```python
from build123d import *

# Parameters (mm, degrees)
SKETCH1_W               = 42.62295082
SKETCH1_H               = 50
SKETCH1_R               = 2.677018134
BOSS_EXTRUDE1_DEPTH     = 20
SKETCH2_R               = 11
CUT_EXTRUDE2_DEPTH      = 11
SKETCH3_R               = 1.75
CUT_EXTRUDE3_DEPTH      = 10
CUT_EXTRUDE6_START      = -5
CUT_EXTRUDE6_DEPTH      = 34.460095998
SKETCH30_W              = 42.62295082
SKETCH30_H              = 20
BOSS_EXTRUDE8_DEPTH     = 20.23
SKETCH10_W              = 42.62295082
SKETCH10_H              = 16
BOSS_EXTRUDE2_DEPTH     = 20
SKETCH14_W              = 6
SKETCH14_H              = 13
CUT_EXTRUDE7_DEPTH      = 78.238778062
BOSS_EXTRUDE3_DEPTH     = 8
CUT_EXTRUDE9_DEPTH      = 8
SKETCH18_W              = 0.9
SKETCH18_H              = 4
SKETCH18_W_2            = 1.8
CUT_EXTRUDE10_DEPTH     = 10.2
CUT_EXTRUDE8_DEPTH      = 71.769170482
CUT_EXTRUDE8_DEPTH_BACK = 71.769170482
SKETCH15_R              = 1
CUT_EXTRUDE5_DEPTH      = 82.374415455
CUT_EXTRUDE5_DEPTH_BACK = 50
SKETCH6_W               = 9.034037672
SKETCH6_H               = 5.5
SKETCH20_W              = 8
SKETCH20_H              = 20
BOSS_EXTRUDE5_DEPTH     = 13
SKETCH21_W              = 8
SKETCH21_H              = 6
CUT_EXTRUDE11_DEPTH     = 13
SKETCH22_R              = 1
CUT_EXTRUDE12_DEPTH     = 71.769170482
SKETCH24_W              = 50.62295082
SKETCH24_H              = 5
BOSS_EXTRUDE6_DEPTH     = 15
SKETCH25_W              = 50.62295082
SKETCH25_H              = 15
BOSS_EXTRUDE7_DEPTH     = 15
SKETCH26_R              = 1
CUT_EXTRUDE13_DEPTH     = 10
SKETCH27_W              = 4
SKETCH27_H              = 1.8
CUT_EXTRUDE14_DEPTH     = 10.2
SKETCH29_W              = 20
SKETCH29_H              = 3.2
CUT_EXTRUDE15_DEPTH     = 9


with BuildPart() as part:
    # Sketch1 → Boss-Extrude1 (new body)
    with BuildSketch(Plane.XY):
        Rectangle(SKETCH1_W, SKETCH1_H)
        with Locations((-13, -15.25)):
            Circle(SKETCH1_R, mode=Mode.SUBTRACT)
        with Locations(Location((13, -15.25, 0), (0, 0, 180))):
            Circle(SKETCH1_R, mode=Mode.SUBTRACT)
        with Locations((13, 15.25)):
            Circle(SKETCH1_R, mode=Mode.SUBTRACT)
        with Locations(Location((-13, 15.25, 0), (0, 0, 180))):
            Circle(SKETCH1_R, mode=Mode.SUBTRACT)
    extrude(amount=BOSS_EXTRUDE1_DEPTH)

    # Sketch2 → Cut-Extrude2 (cut)
    with BuildSketch(Plane.XY):
        Circle(SKETCH2_R)
    extrude(amount=CUT_EXTRUDE2_DEPTH, mode=Mode.SUBTRACT)

    # Sketch3 → Cut-Extrude3 (cut)
    with BuildSketch(Plane(origin=(0, 0, 0), x_dir=(-1, 0, 0), z_dir=(0, 0, -1))):
        with Locations((-15, 0)):
            Circle(SKETCH3_R)
        with Locations(Location((15, 0, 0), (0, 0, 180))):
            Circle(SKETCH3_R)
    extrude(amount=-CUT_EXTRUDE3_DEPTH, mode=Mode.SUBTRACT)

    # Sketch9 → Cut-Extrude6 (cut, through all)
    with BuildSketch(Plane(origin=(0, 0, 0), x_dir=(-1, 0, 0), z_dir=(0, 0, -1)).offset(CUT_EXTRUDE6_START)):
        Polygon((-15, 3.175426481), (-17.75, 1.58771324), (-17.75, -1.58771324), (-15, -3.175426481), (-12.25, -1.58771324), (-12.25, 1.58771324), align=None)
        Polygon((12.25, 1.58771324), (15, 3.175426481), (17.75, 1.58771324), (17.75, -1.58771324), (15, -3.175426481), (12.25, -1.58771324), align=None)
    extrude(amount=-CUT_EXTRUDE6_DEPTH, mode=Mode.SUBTRACT)

    # Sketch30 → Boss-Extrude8 (add)
    with BuildSketch(Plane.XZ.offset(25)):
        with Locations((0, 10)):
            Rectangle(SKETCH30_W, SKETCH30_H)
    extrude(amount=BOSS_EXTRUDE8_DEPTH)

    # Sketch10 → Boss-Extrude2 (add)
    with BuildSketch(Plane.XY):
        with Locations((0, -53.23)):
            Rectangle(SKETCH10_W, SKETCH10_H)
    extrude(amount=BOSS_EXTRUDE2_DEPTH)

    # Sketch14 → Cut-Extrude7 (cut, through all)
    with BuildSketch(Plane.ZY.offset(21.31147541)):
        with Locations((8, -54.73)):
            Rectangle(SKETCH14_W, SKETCH14_H)
    extrude(amount=-CUT_EXTRUDE7_DEPTH, mode=Mode.SUBTRACT)

    # Sketch16 → Boss-Extrude3 (add)
    with BuildSketch(Plane(origin=(21.31147541, 0, 0), x_dir=(0, 0, -1), z_dir=(1, 0, 0))):
        Polygon((-10, 25), (-10, -48.23), (-5, -48.23), (0, -48.23), (0, 25), align=None)
        Polygon((-11, -48.23), (-10, -48.23), (-10, 25), (-20, 25), (-20, -48.23), align=None)
    extrude(amount=BOSS_EXTRUDE3_DEPTH)

    # Sketch17 → Cut-Extrude9 (cut)
    with BuildSketch(Plane(origin=(29.31147541, 0, 0), x_dir=(0, 0, -1), z_dir=(1, 0, 0))):
        with BuildLine():
            ThreePointArc((-10, 7.56), (-11.175, 6.385), (-10, 5.21))
            Line((-10, 5.21), (-10, 7.56))
        make_face()
        with BuildLine():
            Line((-10, 7.56), (-10, 5.21))
            ThreePointArc((-10, 5.21), (-9.169149532, 5.554149532), (-8.825, 6.385))
            ThreePointArc((-8.825, 6.385), (-9.169149532, 7.215850468), (-10, 7.56))
        make_face()
        with BuildLine():
            ThreePointArc((-10, -28.44), (-11.175, -29.615), (-10, -30.79))
            Line((-10, -30.79), (-10, -28.44))
        make_face()
        with BuildLine():
            Line((-10, -28.44), (-10, -30.79))
            ThreePointArc((-10, -30.79), (-9.169149532, -30.445850468), (-8.825, -29.615))
            ThreePointArc((-8.825, -29.615), (-9.169149532, -28.784149532), (-10, -28.44))
        make_face()
    extrude(amount=-CUT_EXTRUDE9_DEPTH, mode=Mode.SUBTRACT)

    # Sketch18 → Cut-Extrude10 (cut)
    with BuildSketch(Plane(origin=(0, 0, 0), x_dir=(-1, 0, 0), z_dir=(0, 0, -1))):
        with Locations((-24.86147541, 6.385)):
            Rectangle(SKETCH18_W, SKETCH18_H)
        with Locations((-25.76147541, 6.385)):
            Rectangle(SKETCH18_W, SKETCH18_H)
        with Locations((-25.31147541, -29.615)):
            Rectangle(SKETCH18_W_2, SKETCH18_H)
    extrude(amount=-CUT_EXTRUDE10_DEPTH, mode=Mode.SUBTRACT)

    # Sketch15 → Cut-Extrude8 (cut, two sides: drawn at the far end of the back side and taken through both)
    with BuildSketch(Plane(origin=(0, 0, 0), x_dir=(-1, 0, 0), z_dir=(0, 0, -1)).offset(-CUT_EXTRUDE8_DEPTH_BACK)):
        with Locations(Location((16.31147541, -58.03, 0), (0, 0, 180))):
            Circle(SKETCH15_R)
        with Locations((16.31147541, -51.43)):
            Circle(SKETCH15_R)
    extrude(amount=CUT_EXTRUDE8_DEPTH + CUT_EXTRUDE8_DEPTH_BACK, mode=Mode.SUBTRACT)

    # Sketch6 → Cut-Extrude5 (cut, two sides: drawn at the far end of the back side and taken through both)
    with BuildSketch(Plane.XZ.offset(48.23).offset(-CUT_EXTRUDE5_DEPTH_BACK)):
        with Locations((0, 13.75)):
            Rectangle(SKETCH6_W, SKETCH6_H)
    extrude(amount=CUT_EXTRUDE5_DEPTH + CUT_EXTRUDE5_DEPTH_BACK, mode=Mode.SUBTRACT)

    # Sketch20 → Boss-Extrude5 (add)
    with BuildSketch(Plane(origin=(0, -48.23, 0), x_dir=(-1, 0, 0), z_dir=(0, -1, 0))):
        with Locations((-25.31147541, -10)):
            Rectangle(SKETCH20_W, SKETCH20_H)
    extrude(amount=BOSS_EXTRUDE5_DEPTH)

    # Sketch21 → Cut-Extrude11 (cut)
    with BuildSketch(Plane(origin=(0, -61.23, 0), x_dir=(-1, 0, 0), z_dir=(0, -1, 0))):
        with Locations((-25.31147541, -8)):
            Rectangle(SKETCH21_W, SKETCH21_H)
    extrude(amount=-CUT_EXTRUDE11_DEPTH, mode=Mode.SUBTRACT)

    # Sketch22 → Cut-Extrude12 (cut, through all)
    with BuildSketch(Plane(origin=(0, 0, 0), x_dir=(-1, 0, 0), z_dir=(0, 0, -1))):
        with Locations((-24.31147541, -58.03)):
            Circle(SKETCH22_R)
        with Locations((-24.31147541, -51.43)):
            Circle(SKETCH22_R)
    extrude(amount=-CUT_EXTRUDE12_DEPTH, mode=Mode.SUBTRACT)

    # Sketch24 → Boss-Extrude6 (add)
    with BuildSketch(Plane.XZ.offset(61.23)):
        with Locations((4, 2.5)):
            Rectangle(SKETCH24_W, SKETCH24_H)
    extrude(amount=BOSS_EXTRUDE6_DEPTH)

    # Sketch25 → Boss-Extrude7 (add)
    with BuildSketch(Plane.XY.offset(5)):
        with Locations((4, -68.73)):
            Rectangle(SKETCH25_W, SKETCH25_H)
    extrude(amount=BOSS_EXTRUDE7_DEPTH)

    # Sketch26 → Cut-Extrude13 (cut)
    with BuildSketch(Plane.XZ.offset(76.23)):
        with BuildLine():
            ThreePointArc((-15, 10), (-14, 9), (-13, 10))
            Line((-13, 10), (-15, 10))
        make_face()
        with BuildLine():
            Line((-15, 10), (-13, 10))
            ThreePointArc((-13, 10), (-14, 11), (-15, 10))
        make_face()
        with Locations(Location((22, 10, 0), (0, 0, 270))):
            Circle(SKETCH26_R)
    extrude(amount=-CUT_EXTRUDE13_DEPTH, mode=Mode.SUBTRACT)

    # Sketch27 → Cut-Extrude14 (cut)
    with BuildSketch(Plane(origin=(0, 0, 0), x_dir=(-1, 0, 0), z_dir=(0, 0, -1))):
        with Locations((-22.00147541, -72.23)):
            Rectangle(SKETCH27_W, SKETCH27_H)
        with Locations((14.00147541, -72.23)):
            Rectangle(SKETCH27_W, SKETCH27_H)
    extrude(amount=-CUT_EXTRUDE14_DEPTH, mode=Mode.SUBTRACT)

    # Sketch29 → Cut-Extrude15 (cut)
    with BuildSketch(Plane.XY.offset(20)):
        with Locations((4, -49.83)):
            Rectangle(SKETCH29_W, SKETCH29_H)
        Polygon((-6, -51.43), (-6, -53.105302663), (4, -54.73), (14, -53.105302663), (14, -51.43), align=None)
        Polygon((4, -54.73), (-6, -53.105302663), (-6, -56.354697337), align=None)
        with Locations((4, -59.63)):
            Rectangle(SKETCH29_W, SKETCH29_H)
        Polygon((14, -56.354697337), (4, -54.73), (-6, -56.354697337), (-6, -58.03), (14, -58.03), align=None)
        Polygon((14, -53.105302663), (4, -54.73), (14, -56.354697337), align=None)
    extrude(amount=-CUT_EXTRUDE15_DEPTH, mode=Mode.SUBTRACT)


solid = part.part
```
Geometry: final body of the model. Coordinates: model frame, mm. A direction names the side the tool comes from. Coordinates: 2 decimals unless noted, no trailing zeros. Order: outer loops, then holes, each group sorted by start corner. A loop starts at its lowest first (then second) coordinate and runs counter-clockwise, first axis right, second up. Notation, with made-up numbers: (24.5, 17.5) -> (78.5, 17.5) arc R28 cw to (78.5, 43.5) -> close; hole circle Ø3 at (-6, 61.25). An arc over 180 degrees is marked (long way). Write each question's results on one line, items separated by ' | '. Start each with the question number.
1) Set-up query: faces 3 (the cylindrical face through (-13.46, -71.3, 10.84)), 4 (the flat face through (22, -71.33, 5)), 5 (the flat face through (12.25, 0, 12)). Return all of +Z, -Z, +X, -X, +Y, -Y with unobstructed straight access to the full face (end or side cutting, diameter ignored); none if empty.
2) First-contact query: pin 1 (0.5 mm diameter, centred on x = 21, y = -72.5, fed in from -Z). Flat tip, straight axial feed; report the tip coordinate or a pass-through.
3) Mould query, pull axis Y, two halves, no side actions, for faces 1 (the flat face through (0, 3, 11)), 2 (the flat face through (29.311, -26, 10)). Classes: released by +Y, released by -Y, zero draft, split by the parting line, or undercut.
4) Cut plane C-C, the plane y = -39. Output: boundary loops of the cut face in (x, z).
5) Material intervals for line 1 along Y through (x, z) = (13, 2.5); line 2 along Y through (x, z) = (-13, 7.5); line 3 along Z through (x, y) = (-0.5, -31), sorted ascending.
6) Cut plane B-B, the plane x = 0. Output: boundary loops of the cut face in (y, z).
7) Cut plane A-A, the plane z = 2.25. State how many separate pieces and enclosed holes the cut face has, and give its area (3 significant figures).
Checks:
1) face 3: -Y | face 4: -Z | face 5: +Z
2) pin 1: z = 10.2
3) face 1: undercut | face 2: zero draft
4) outline: (-21.31, 0) -> (29.31, 0) -> (29.31, 20) -> (-21.31, 20) -> close; hole (-4.52, 11) -> (4.52, 11) -> (4.52, 16.5) -> (-4.52, 16.5) -> close
5) line 1: -76.23 to -17.93, -12.57 to 12.57, 17.93 to 25 | line 2: -76.23 to -73.13, -71.33 to -61.23, -48.23 to -17.93, -12.57 to -2.02, 2.02 to 12.57, 17.93 to 25 | line 3: 0 to 11, 16.5 to 20
6) outline: (-76.23, 0) -> (-11, 0) -> (-11, 11) -> (-48.23, 11) -> (-48.23, 5) -> (-61.23, 5) -> (-61.23, 20) -> (-76.23, 20) -> close; (-48.23, 16.5) -> (1.77, 16.5) -> (1.77, 11) -> (11, 11) -> (11, 0) -> (25, 0) -> (25, 20) -> (-48.23, 20) -> close
7) separate pieces: 1 | enclosed holes: 15 | area: 4,590 mm^2
